Design review of the part shown in the three views and the two pictorial views. Dimensions are in mm from the part's minimum x, y and z. Coordinates: 2 decimals unless noted, no trailing zeros. One line per item, written item: value. Start each with the question number.
1. Insertion check: pin 1 (5 mm diameter, centred on y = 105, z = 18, fed in from +X); pin 2 (3 mm diameter, centred on y = 104, z = 19, fed in from -X). Each pin has a flat end and moves straight along its axis. Give the tip position at first contact, or say it passes through.
2. For probe 1 along Z at (x, y) = (163.25, 105); probe 2 along Y at (x, z) = (137.5, 42), list the stretches that pass through material, from the lowest coordinate up.
3. Draft analysis for pull direction Z (two halves, no side actions). For the marked faces 1, 2 and 3, state which applies: pulls with the +Z half, pulls with the -Z half, needs draft (parallel to the pull), parting line crosses it, or undercut.
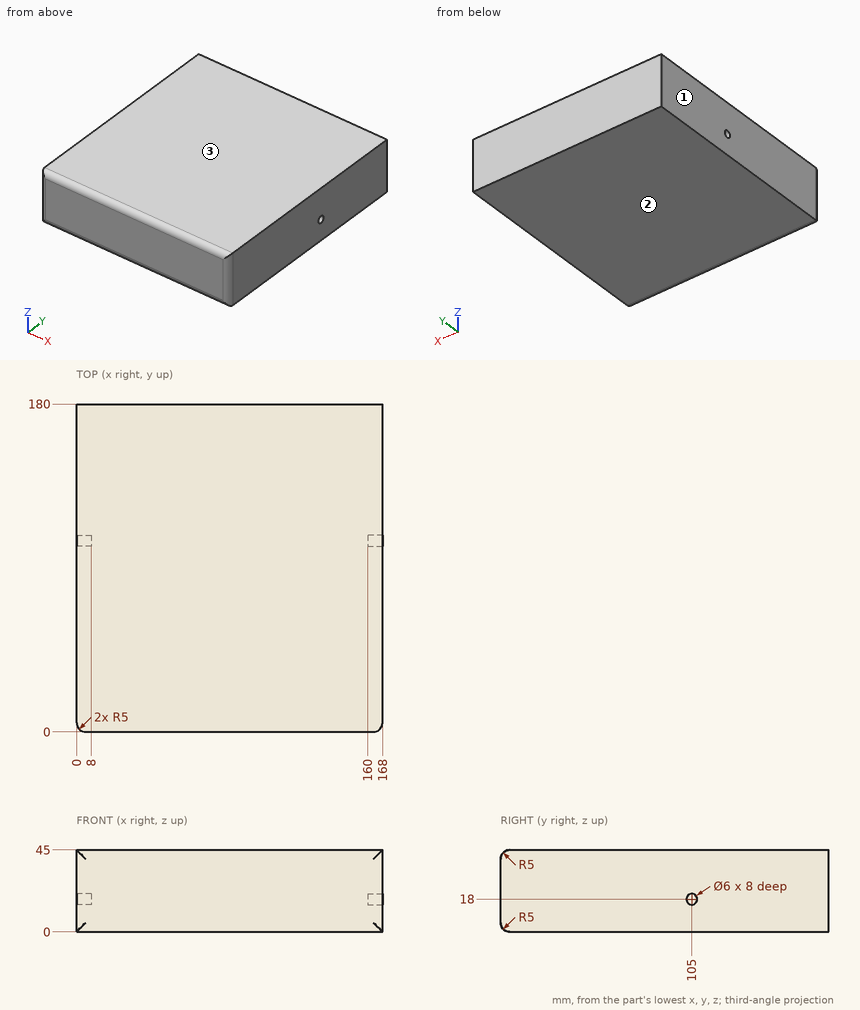
Worked answers:
1. pin 1: stops at x = 160
1. pin 2: stops at x = 8
2. probe 1: z = 0 to 15, 21 to 45
2. probe 2: y = 0.42 to 180
3. face 1: needs draft
3. face 2: pulls with the -Z half
3. face 3: pulls with the +Z half
